Check sheet for the modelled part. Datum: model origin and axes. Units: mm. Give positions to 0.01 mm unless a question says otherwise; leave off trailing zeros. Write each loop counter-clockwise with the first axis right and the second up, starting at its lowest first coordinate (ties: lowest second). Pieces come first, ordered by that corner, then holes. Notation, with made-up numbers: M 74,19.5 L 115,19.5 A29 cw 115,57.5 Z; hole C 15.5,-32 d6. An arc over 180 degrees is marked long. Write item = value, one per line. Start each with the question number.
1) Sectioned sample at A-A, the plane z = 9.5. Record the cut outline in (x, y), then the cut area to 3 significant figures.
2) Gauge pin test, flat ends, axial feed: pin 1 (6.5 mm diameter, centred on x = 0, z = 0, fed in from -Y); pin 2 (0.6 mm diameter, centred on x = 12, y = 1.5, fed in from -Z). Record the tip position at first contact, or that the pin passes through.
3) Sectioned sample at B-B, the plane x = 8. Record the cut outline in (y, z).
4) Sectioned sample at D-D, the plane z = 5.5. Record the cut outline in (x, y).
5) Scan lines: L1, parallel to X at y = 1.85, z = 0; L2, parallel to Z at x = 0, y = 1.35; L3, parallel to X at y = 0.95, z = -9.5. Record each from-to range of solid material in increasing order.
6) Sectioned sample at C-C, the plane y = 0.35. Count the separate pieces of the cut face and the enclosed holes in it, then the cut area to 3 significant figures.
from build123d import *

# Parameters (mm, degrees)
CROQUIS1_R              = 4
CROQUIS1_R_2            = 1.5
SALIENTE_EXTRUIR1_DEPTH = 2


with BuildPart() as part:
    # Croquis1 → Saliente-Extruir1 (new body)
    with BuildSketch(Plane(origin=(0, 0, 0), x_dir=(1, 0, 0), z_dir=(0, 1, 0))):
        with BuildLine():
            Line((16.6, 3.5), (8.5, 3.5))
            ThreePointArc((8.5, 3.5), (4.964466094, 4.964466094), (3.5, 8.5))
            Line((3.5, 8.5), (3.5, 16.6))
            ThreePointArc((3.5, 16.6), (2.504163056, 19.004163056), (0.1, 20))
            Line((0.1, 20), (-0.1, 20))
            ThreePointArc((-0.1, 20), (-2.504163056, 19.004163056), (-3.5, 16.6))
            Line((-3.5, 16.6), (-3.5, 8.5))
            ThreePointArc((-3.5, 8.5), (-4.964466094, 4.964466094), (-8.5, 3.5))
            Line((-8.5, 3.5), (-16.6, 3.5))
            ThreePointArc((-16.6, 3.5), (-19.004163056, 2.504163056), (-20, 0.1))
            Line((-20, 0.1), (-20, -0.1))
            ThreePointArc((-20, -0.1), (-19.004163056, -2.504163056), (-16.6, -3.5))
            Line((-16.6, -3.5), (-8.5, -3.5))
            ThreePointArc((-8.5, -3.5), (-4.964466094, -4.964466094), (-3.5, -8.5))
            Line((-3.5, -8.5), (-3.5, -16.6))
            ThreePointArc((-3.5, -16.6), (-2.504163056, -19.004163056), (-0.1, -20))
            Line((-0.1, -20), (0.1, -20))
            ThreePointArc((0.1, -20), (2.504163056, -19.004163056), (3.5, -16.6))
            Line((3.5, -16.6), (3.5, -8.5))
            ThreePointArc((3.5, -8.5), (4.964466094, -4.964466094), (8.5, -3.5))
            Line((8.5, -3.5), (16.6, -3.5))
            ThreePointArc((16.6, -3.5), (19.004163056, -2.504163056), (20, -0.1))
            Line((20, -0.1), (20, 0.1))
            ThreePointArc((20, 0.1), (19.004163056, 2.504163056), (16.6, 3.5))
        make_face()
        Circle(CROQUIS1_R, mode=Mode.SUBTRACT)
        with Locations((0, 9.5)):
            Circle(CROQUIS1_R_2, mode=Mode.SUBTRACT)
        with Locations((0, 16.25)):
            Circle(CROQUIS1_R_2, mode=Mode.SUBTRACT)
        with Locations((0, -9.5)):
            Circle(CROQUIS1_R_2, mode=Mode.SUBTRACT)
        with Locations((0, -16.25)):
            Circle(CROQUIS1_R_2, mode=Mode.SUBTRACT)
        with Locations((8, 0)):
            Circle(CROQUIS1_R_2, mode=Mode.SUBTRACT)
        with Locations((16.25, 0)):
            Circle(CROQUIS1_R_2, mode=Mode.SUBTRACT)
        with Locations((-16.25, 0)):
            Circle(CROQUIS1_R_2, mode=Mode.SUBTRACT)
        with Locations((-8, 0)):
            Circle(CROQUIS1_R_2, mode=Mode.SUBTRACT)
    extrude(amount=SALIENTE_EXTRUIR1_DEPTH)


solid = part.part
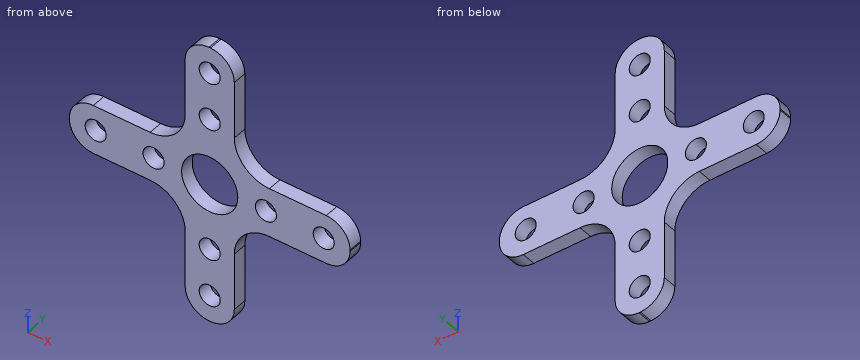
Data:
q1.outline = M -3.5,0 L -1.5,0 L -1.5,2 L -3.5,2 Z; M 1.5,0 L 3.5,0 L 3.5,2 L 1.5,2 Z
q1.area = 8.00 mm2
q2.pin_1 = through
q2.pin_2 = -3.5
q3.outline = M 0,-3.53 L 2,-3.53 L 2,-1.5 L 0,-1.5 Z; M 0,1.5 L 2,1.5 L 2,3.53 L 0,3.53 Z
q4.outline = M -4.5,0 L 4.5,0 L 4.5,2 L -4.5,2 Z
q5.L1 = -20 to -17.75, -14.75 to -9.5, -6.5 to -4, 4 to 6.5, 9.5 to 14.75, 17.75 to 20
q5.L2 = -20 to -17.75, -14.75 to -11, -8 to -4, 4 to 8, 11 to 14.75, 17.75 to 20
q5.L3 = -3.5 to -1.5, 1.5 to 3.5
q6.separate_pieces = 1
q6.enclosed_holes = 9
q6.area = 406 mm2
